Build history of the part. All positions in model axes, mm. Coordinates: 2 decimals unless noted, no trailing zeros. Write each loop counter-clockwise with the first axis right and the second up, starting at its lowest first coordinate (ties: lowest second). Pieces come first, ordered by that corner, then holes. Notation, with made-up numbers: (36.25, 64.25) -> (68.25, 64.25) arc R27 cw to (68.25, 100.25) -> close; hole circle Ø9 at (-35, 12). An arc over 180 degrees is marked (long way). Write each question's results on one line, items separated by ' | '. Start each with the question number.
Q1. Drill centre lines: line 1 (X direction, y = 48, z = 5.5); line 2 (X direction, y = -77, z = 4.5); line 3 (Y direction, x = -38, z = 10.5). Where is each one in solid material? Low to high.
Q2. Saw through at B-B on y = 47. Give the cut face in (x, z).
Q3. Drop flat-ended pins along their axis: pin 1 Ø5 at (x, z) = (43, 18.5) entering from +Y; pin 2 Ø10 at (y, z) = (73.5, 16) entering from -X; pin 3 Ø1 at (y, z) = (48.5, 12) entering from +X. Give the stop position or say it passes through.
Q4. Saw through at A-A on z = 15.5. Give the cut face in (x, y).
Q5. Saw through at C-C on x = -45.5. Give the cut face in (y, z).
from build123d import *

# Parameters (mm, degrees)
F1_DEPTH = 25.4


with BuildPart() as f1:
    # F0 (on Top) → F1 (new body)
    with BuildSketch(Plane.XY):
        with BuildLine():
            ThreePointArc((116.3974231574, -50.7999988418), (124.3211018713, -25.94732413), (127, 0))
            ThreePointArc((127, 0), (121.171970747, 38.0309545671), (104.2227794443, 72.5714285714))
            ThreePointArc((104.2227794443, 72.5714285714), (0, 127), (-104.2227794443, 72.5714285714))
            ThreePointArc((-104.2227794443, 72.5714285714), (-126.3860979139, 12.4721391145), (-116.3974224673, -50.8000004228))
            ThreePointArc((-116.3974224673, -50.8000004228), (-83.5987115374, 32.7987112337), (0, 0))
            ThreePointArc((0, 0), (71.1723737002, 36.7605508711), (121.6987113259, -25.4))
            ThreePointArc((121.6987113259, -25.4), (120.3592623261, -38.3736617557), (116.3974231574, -50.7999988418))
        make_face()
        with BuildLine():
            ThreePointArc((0, 0), (-83.5987115374, 32.7987112337), (-116.3974224673, -50.8000004228))
            ThreePointArc((-116.3974224673, -50.8000004228), (-101.6129668627, -71.7406130321), (-79.7537895948, -85.1296291703))
            ThreePointArc((-79.7537895948, -85.1296291703), (-33.0925403585, -83.7260677515), (0, -50.8))
            ThreePointArc((0, -50.8), (-5.3012886741, -25.4), (0, 0))
        make_face()
        with BuildLine():
            ThreePointArc((5.3012886741, -25.4), (3.9618395452, -12.4263376257), (0, 0))
            ThreePointArc((0, 0), (-5.3012886741, -25.4), (0, -50.8))
            ThreePointArc((0, -50.8), (3.9618395452, -38.3736623743), (5.3012886741, -25.4))
        make_face()
        with BuildLine():
            ThreePointArc((79.7537895948, -85.1296291703), (101.6129674921, -71.7406124424), (116.3974231574, -50.7999988418))
            ThreePointArc((116.3974231574, -50.7999988418), (120.3592623261, -38.3736617557), (121.6987113259, -25.4))
            ThreePointArc((121.6987113259, -25.4), (71.1723737002, 36.7605508711), (0, 0))
            ThreePointArc((0, 0), (3.9618395452, -12.4263376257), (5.3012886741, -25.4))
            ThreePointArc((5.3012886741, -25.4), (3.9618395452, -38.3736623743), (0, -50.8))
            ThreePointArc((0, -50.8), (33.0925403585, -83.7260677515), (79.7537895948, -85.1296291703))
        make_face()
        with BuildLine():
            ThreePointArc((-79.7537895948, -85.1296291703), (0, -99.0800012402), (79.7537895948, -85.1296291703))
            ThreePointArc((79.7537895948, -85.1296291703), (33.0925403585, -83.7260677515), (0, -50.8))
            ThreePointArc((0, -50.8), (-33.0925403585, -83.7260677515), (-79.7537895948, -85.1296291703))
        make_face()
        with BuildLine():
            ThreePointArc((-104.2227794443, 72.5714285714), (0, 127), (104.2227794443, 72.5714285714))
            ThreePointArc((104.2227794443, 72.5714285714), (69.1473175054, 138.2082566307), (50.314445249, 210.2068965517))
            ThreePointArc((50.314445249, 210.2068965517), (50.678465933, 206.711850036), (50.8, 203.2))
            ThreePointArc((50.8, 203.2), (-3.511850036, 152.521534067), (-50.314445249, 210.2068965517))
            ThreePointArc((-50.314445249, 210.2068965517), (-69.1473175054, 138.2082566307), (-104.2227794443, 72.5714285714))
        make_face()
        with BuildLine():
            ThreePointArc((50.8, 203.2), (50.678465933, 206.711850036), (50.314445249, 210.2068965517))
            ThreePointArc((50.314445249, 210.2068965517), (0, 254), (-50.314445249, 210.2068965517))
            ThreePointArc((-50.314445249, 210.2068965517), (-3.511850036, 152.521534067), (50.8, 203.2))
        make_face()
    extrude(amount=F1_DEPTH)


solid = f1.part
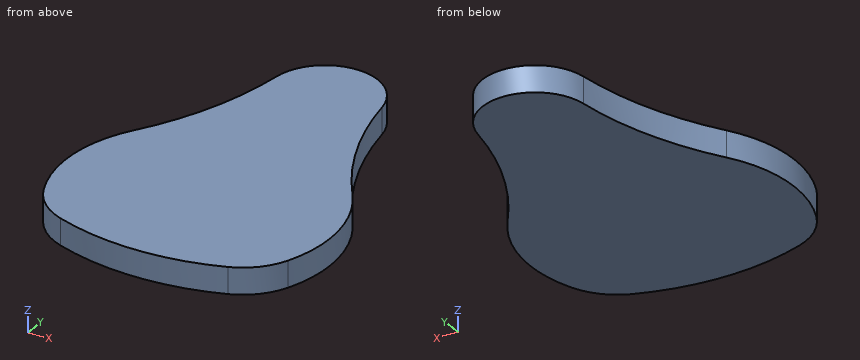
Returned:
1) line 1: x = -117.58 to 117.58 | line 2: x = -95.21 to 95.21 | line 3: y = -95.99 to 236.91
2) outline: (-117.98, 0) -> (117.98, 0) -> (117.98, 25.4) -> (-117.98, 25.4) -> close
3) pin 1: stops at y = 233.87 | pin 2: stops at x = -106.94 | pin 3: stops at x = 117.58
4) outline: (-116.4, -50.8) arc R63.5 ccw to (-79.75, -85.13) arc R234.95 ccw to (79.75, -85.13) arc R63.5 ccw to (116.4, -50.8) arc R127 ccw to (104.22, 72.57) arc R317.5 cw to (50.31, 210.21) arc R50.8 ccw to (-50.31, 210.21) arc R317.5 cw to (-104.22, 72.57) arc R127 ccw to start
5) outline: (-94.63, 0) -> (225.79, 0) -> (225.79, 25.4) -> (-94.63, 25.4) -> close
